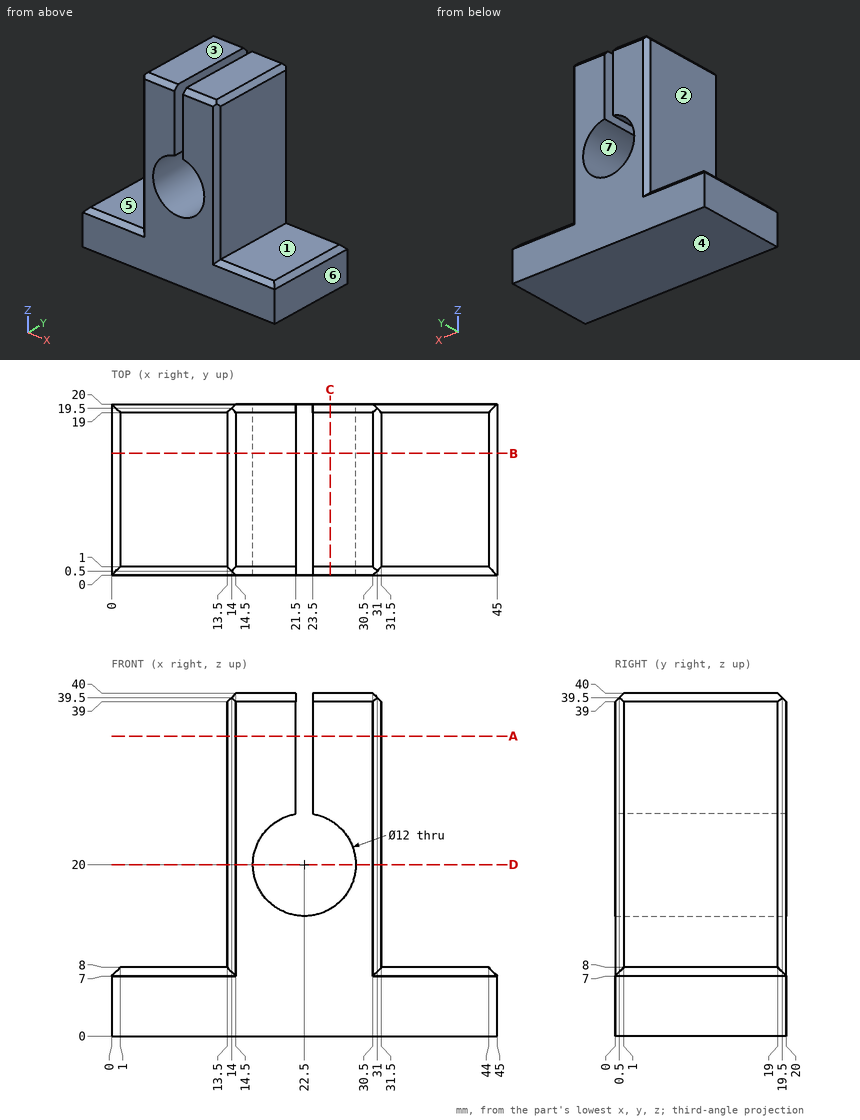
For this review, use the dimensioned drawing (mm, ordinates from the lowest corner) and the shaded views. A direction names the side the tool comes from. Give positions to 0.01 mm unless a question says otherwise; leave off trailing zeros. Order: outer loops, then holes, each group sorted by start corner. A loop starts at its lowest first (then second) coordinate and runs counter-clockwise, first axis right, second up. Notation, with made-up numbers: (53.25, 12) - (92.25, 12) arc R14 ccw to (92.25, 22) - close; hole circle Ø4 at (58, -38.75). An arc over 180 degrees is marked (long way). Use CSV: the item, a comma, the result in double quotes. Start each with the question number.
Q1. We need section D-D, the plane z = 20. Write out the cut boundary in (x, y).
Q2. We need section B-B, the plane y = 14.25. Write out the cut boundary in (x, z), and give its area (3 significant figures).
Q3. Tool access review of the marked faces 1, 2 and 3: name each direction out of +Z, -Z, +X, -X, +Y, -Y from which nothing blocks a thin tool from reaching the whole face with its end or side.
Q4. To check wall thickness, follow line 1 along X through (y, z) = (7.5, 20); line 2 along X through (y, z) = (17, 32.5); line 3 along Z through (x, y) = (22.5, 5). State the ranges of each line that lie inside material, in increasing order. Write a range as [from, to].
Q5. The part is to be moulded in two halves that separate along Z. For the marked faces 4, 5, 6 and 7, say which applies: +Z half, -Z half, draft (parallel to the pull), parting line (faces both ways), or undercut.
Q6. We need section A-A, the plane z = 35. Write out the cut boundary in (x, y), and give its area (3 significant figures).
Q7. We need section C-C, the plane x = 25.5. Write out the cut boundary in (y, z).
Q8. Clearance check with flat-ended pins moving along their axes: pin 1 Ø3 at (y, z) = (8, 16.5) entering from +X; pin 2 Ø11.5 at (y, z) = (11, 30) entering from -X; pin 3 Ø2 at (x, y) = (5.5, 7.5) entering from +Z. State where each tip first meets the part, or that it passes through.
Outcome:
1,outline,"(13.5, 1) - (14.5, 0) - (16.5, 0) - (16.5, 20) - (14.5, 20) - (13.5, 19) - close; (28.5, 0) - (30.5, 0) - (31.5, 1) - (31.5, 19) - (30.5, 20) - (28.5, 20) - close"
2,outline,"(0, 0) - (45, 0) - (45, 7) - (44, 8) - (31.5, 8) - (31.5, 39) - (30.5, 40) - (23.5, 40) - (23.5, 25.92) arc R6 cw (long way) to (21.5, 25.92) - (21.5, 40) - (14.5, 40) - (13.5, 39) - (13.5, 8) - (1, 8) - (0, 7) - close"
2,area,"793 mm^2"
3,face 1,"+Z, +X, +Y, -Y"
3,face 2,"+Z, -X, +Y, -Y"
3,face 3,"+Z, +X, -X, +Y, -Y"
4,line 1,"x = [13.5, 16.5], [28.5, 31.5]"
4,line 2,"x = [13.5, 21.5], [23.5, 31.5]"
4,line 3,"z = [0, 14]"
5,face 4,"-Z half"
5,face 5,"+Z half"
5,face 6,"draft"
5,face 7,"undercut"
6,outline,"(13.5, 1) - (14.5, 0) - (21.5, 0) - (21.5, 20) - (14.5, 20) - (13.5, 19) - close; (23.5, 0) - (30.5, 0) - (31.5, 1) - (31.5, 19) - (30.5, 20) - (23.5, 20) - close"
6,area,"318 mm^2"
7,outline,"(0, 0) - (20, 0) - (20, 14.8) - (0, 14.8) - close; (0, 25.2) - (20, 25.2) - (20, 39) - (19, 40) - (1, 40) - (0, 39) - close"
8,pin 1,"stops at x = 31.5"
8,pin 2,"stops at x = 13.5"
8,pin 3,"stops at z = 8"
